from build123d import *

# Parameters (mm, degrees)
F0_W     = 270
F0_H     = 30
F1_DEPTH = 6
F3_D     = 4.2
F5_D     = 3.3


with BuildPart() as f1:
    # F0 (on Front) → F1 (new body)
    with BuildSketch(Plane.XZ):
        with Locations((135, 15)):
            Rectangle(F0_W, F0_H)
    extrude(amount=F1_DEPTH)

    # F3 (through all)
    with Locations(Plane(origin=(0, 0, 0), x_dir=(1, 0, 0), z_dir=(0, 1, 0))):
        with Locations((66, -15), (82, -24), (82, -6), (204, -15), (188, -24), (188, -6)):
            Hole(F3_D / 2)

    # F5 (through all)
    with Locations(Plane(origin=(0, 0, 0), x_dir=(1, 0, 0), z_dir=(0, 1, 0))):
        with Locations((41, -24), (69, -24), (69, -6), (41, -6), (201, -24), (229, -24), (229, -6), (201, -6)):
            Hole(F5_D / 2)


solid = f1.part
Model file for the job. Use its own axes, mm. Round coordinates to 2 decimals unless told otherwise and drop trailing zeros.
(1) Band-saw the part on A-A (y = -2.45). Give the number of separate pieces and of enclosed holes in the cut face, then the cut area to 3 significant figures.
(2) Drill centre lines: line 1 (Z direction, x = 188, y = -3); line 2 (Z direction, x = 201, y = -4.7); line 3 (X direction, y = -1.35, z = 15). Where is each one in solid material? Low to high.
(3) Pull direction Z, two halves, no side cores. Call faces 1 (the face through (133, -6, 15)), 2 (the face through (186.06, -3.04, 6.8)), 3 (the face through (133, -3, 30)): released by +Z, released by -Z, zero draft, split by the parting line, or undercut.
Verdict:
1. separate pieces: 1
1. enclosed holes: 14
1. area: 7,950 mm2
2. line 1: z = 0 to 3.9, 8.1 to 21.9, 26.1 to 30
2. line 2: z = 0 to 4.35, 7.65 to 22.35, 25.65 to 30
2. line 3: x = 0 to 63.9, 68.1 to 201.9, 206.1 to 270
3. face 1: zero draft
3. face 2: undercut
3. face 3: released by +Z
